from build123d import *

# Parameters (mm, degrees)
SKETCH1_W                       = 82.55
SKETCH1_H                       = 57.15
BOSS_EXTRUDE1_DEPTH             = 8.636
FILLET2_R                       = 7.62
FILLET3_R                       = 3.81
SKETCH2_W                       = 63.5
SKETCH2_H                       = 40.64
CUT_EXTRUDE1_DEPTH              = 5.461
SKETCH7_W                       = 68.58
SKETCH7_H                       = 45.72
BOSS_EXTRUDE3_DEPTH             = 5.08
SKETCH8_W                       = 63.5
SKETCH8_H                       = 40.64
CUT_EXTRUDE3_DEPTH              = 5.08
SKETCH5_R                       = 1.016
BOSS_EXTRUDE4_DEPTH             = 12.7
SKETCH4_R                       = 2.25
SKETCH4_W                       = 12.6
SKETCH4_H                       = 5
SKETCH4_W_2                     = 6.604
SKETCH4_H_2                     = 6.604
CUT_EXTRUDE2_DEPTH              = 7.366
FILLET7_R                       = 1.016
FILLET8_R                       = 2.54
SKETCH9_W                       = 12.753817634
SKETCH9_H                       = 4.826
BOSS_EXTRUDE5_DEPTH             = 5.08
FILLET10_R                      = 7.62
FILLET11_R                      = 1.27
FILLET12_R                      = 1.016
F_4_40_TAPPED_HOLE2_D           = 2.2606
F_4_40_TAPPED_HOLE2_DEPTH       = 7.62
F_4_40_TAPPED_HOLE2_CSINK_D     = 4.1148
F_4_40_TAPPED_HOLE2_CSINK_ANGLE = 100
F_4_40_TAPPED_HOLE2_TIP         = 0.679152758


with BuildPart() as part:
    # Sketch1 → Boss-Extrude1 (new body)
    with BuildSketch(Plane(origin=(0, 0, 0), x_dir=(1, 0, 0), z_dir=(0, 1, 0))):
        with Locations((41.275, 28.575)):
            Rectangle(SKETCH1_W, SKETCH1_H)
    extrude(amount=BOSS_EXTRUDE1_DEPTH)

    # Fillet2
    fillet2_edges = [part.edges().sort_by_distance(p)[0] for p in [
        (0, 4.318, -57.15),
        (82.55, 4.318, -57.15),
        (82.55, 4.318, 0),
        (0, 4.318, 0),
    ]]
    fillet(fillet2_edges, radius=FILLET2_R)

    # Fillet3
    fillet3_edges = [part.edges().sort_by_distance(p)[0] for p in [
        (41.275, 0, -57.15),
        (0, 0, -28.575),
        (82.55, 0, -28.575),
        (41.275, 0, 0),
        (2.231846327, 0, -54.918153673),
        (2.231846327, 0, -2.231846327),
        (80.318153673, 0, -2.231846327),
        (80.318153673, 0, -54.918153673),
    ]]
    fillet(fillet3_edges, radius=FILLET3_R)

    # Sketch2 → Cut-Extrude1 (cut)
    with BuildSketch(Plane(origin=(0, 8.636, 0), x_dir=(1, 0, 0), z_dir=(0, 1, 0))):
        with Locations((41.275, 28.575)):
            Rectangle(SKETCH2_W, SKETCH2_H)
    extrude(amount=-CUT_EXTRUDE1_DEPTH, mode=Mode.SUBTRACT)

    # Sketch7 → Boss-Extrude3 (add)
    with BuildSketch(Plane(origin=(0, 8.636, 0), x_dir=(1, 0, 0), z_dir=(0, 1, 0))):
        with Locations((41.275, 28.575)):
            Rectangle(SKETCH7_W, SKETCH7_H)
    extrude(amount=BOSS_EXTRUDE3_DEPTH)

    # Sketch8 → Cut-Extrude3 (cut)
    with BuildSketch(Plane(origin=(0, 13.716, 0), x_dir=(1, 0, 0), z_dir=(0, 1, 0))):
        with Locations((41.275, 28.575)):
            Rectangle(SKETCH8_W, SKETCH8_H)
    extrude(amount=-CUT_EXTRUDE3_DEPTH, mode=Mode.SUBTRACT)

    # Sketch5 → Boss-Extrude4 (add)
    with BuildSketch(Plane(origin=(0, 3.175, 0), x_dir=(1, 0, 0), z_dir=(0, 1, 0))):
        with Locations(Location((17.665, 42.392, 0), (0, 0, 90))):
            Circle(SKETCH5_R)
        with Locations(Location((17.665, 14.732, 0), (0, 0, 90))):
            Circle(SKETCH5_R)
        with Locations(Location((67.945, 42.259, 0), (0, 0, 90))):
            Circle(SKETCH5_R)
        with Locations(Location((67.945, 14.859, 0), (0, 0, 90))):
            Circle(SKETCH5_R)
    extrude(amount=BOSS_EXTRUDE4_DEPTH)

    # Sketch4 → Cut-Extrude2 (cut)
    with BuildSketch(Plane(origin=(0, 3.175, 0), x_dir=(1, 0, 0), z_dir=(0, 1, 0))):
        with Locations(Location((45.641, 18.034, 0), (0, 0, 270))):
            Circle(SKETCH4_R)
        with Locations((60.171, 18.059)):
            Rectangle(SKETCH4_W, SKETCH4_H)
        with Locations((32.983, 18.034)):
            Rectangle(SKETCH4_W_2, SKETCH4_H_2)
    extrude(amount=-CUT_EXTRUDE2_DEPTH, mode=Mode.SUBTRACT)

    # Fillet7
    fillet7_edges = [part.edges().sort_by_distance(p)[0] for p in [
        (17.665, 15.875, -41.376),
        (17.665, 15.875, -13.716),
        (67.945, 15.875, -41.243),
    ]]
    fillet(fillet7_edges, radius=FILLET7_R)

    # Fillet8
    fillet8_edges = [part.edges().sort_by_distance(p)[0] for p in [
        (75.565, 11.176, -51.435),
        (6.985, 11.176, -51.435),
        (6.985, 11.176, -5.715),
        (75.565, 11.176, -5.715),
    ]]
    fillet(fillet8_edges, radius=FILLET8_R)

    # Sketch9 → Boss-Extrude5 (add)
    with BuildSketch(Plane.XY):
        with Locations((41.275, 6.223)):
            Rectangle(SKETCH9_W, SKETCH9_H)
    extrude(amount=BOSS_EXTRUDE5_DEPTH)

    # Fillet10
    # the kernel refuses this fillet: 7.62 mm, written as the material it takes off along each edge
    with BuildSketch(Plane(origin=(47.651908817, -14.150512242, 5.08), x_dir=(0, 0, -1), z_dir=(0, 1, 0)), Plane(origin=(34.898091183, 26.596512242, 5.08), x_dir=(0, 0, -1), z_dir=(0, -1, 0))) as fillet10_piece_1:
        with BuildLine():
            CenterArc((7.62, 7.184204897), FILLET10_R, 180, 70.528779366)
            Line((0, 7.184204897), (-0.1524, 7.184204897))
            Line((-0.1524, 7.184204897), (-0.1524, 0))
            Line((-0.1524, 0), (0, -0.1524))
            ThreePointArc((0, -0.1524), (2.54, -0.1524), (5.0292, -0.143684098))
            Line((5.0292, -0.143684098), (5.08, 0))
        make_face()
    extrude(amount=40.747024484, mode=Mode.SUBTRACT)

    # Fillet11
    fillet11_edges = [part.edges().sort_by_distance(p)[0] for p in [
        (41.275, 13.716, -51.435),
        (75.565, 13.716, -28.575),
        (6.985, 13.716, -28.575),
        (41.275, 13.716, -5.715),
        (7.728948776, 13.716, -50.691051224),
        (7.728948776, 13.716, -6.458948776),
        (74.821051224, 13.716, -6.458948776),
        (74.821051224, 13.716, -50.691051224),
    ]]
    fillet(fillet11_edges, radius=FILLET11_R)

    # Fillet12
    fillet12_edges = [part.edges().sort_by_distance(p)[0] for p in [
        (67.945, 15.875, -13.843),
    ]]
    fillet(fillet12_edges, radius=FILLET12_R)

    # #4-40 Tapped Hole2
    with Locations(Plane(origin=(0, 3.81, 0), x_dir=(-1, 0, 0), z_dir=(0, -1, 0))):
        with Locations((-41.275, -2.518557543)):
            CounterSinkHole(F_4_40_TAPPED_HOLE2_D / 2, F_4_40_TAPPED_HOLE2_CSINK_D / 2, depth=F_4_40_TAPPED_HOLE2_DEPTH, counter_sink_angle=F_4_40_TAPPED_HOLE2_CSINK_ANGLE)
            with Locations((0, 0, -(F_4_40_TAPPED_HOLE2_DEPTH + F_4_40_TAPPED_HOLE2_TIP / 2))):  # 118° drill point
                Cone(0, F_4_40_TAPPED_HOLE2_D / 2, F_4_40_TAPPED_HOLE2_TIP, mode=Mode.SUBTRACT)


solid = part.part
The listing builds one solid part. Answer for the finished solid, in the listing's coordinates (mm). A direction names the side the tool comes from. Give positions to 0.01 mm unless a question says otherwise; leave off trailing zeros. Write each loop counter-clockwise with the first axis right and the second up, starting at its lowest first coordinate (ties: lowest second). Pieces come first, ordered by that corner, then holes.
1) A tool of negligible diameter and unlimited length cuts with its end or side. For faces 4 (the face through (33, 2, -21.336)), 5 (the face through (41, 11, -5.715)), 6 (the face through (7.71, 10.57, -6.48)), 7 (the face through (74.8, 10.57, -6.44)), 8 (the face through (67.64, 8.94, -15.83)), from which of +Z, -Z, +X, -X, +Y, -Y can it reach the whole face along a straight path? Write none if from no direction.
2) For a pull along X with two mould halves and no side action, classify faces 1 (the face through (73.025, 9, -28)), 2 (the face through (0, 6, -28)), 3 (the face through (74.8, 10.57, -50.71)) as pulls with the +X half, pulls with the -X half, needs draft (parallel to the pull), parting line crosses it, or undercut.
3) Section A-A (x = 12.5) is taken. Write down the section's boundary in (y, z) (3 decimals).
4) Find the intervals of material crossed by L1, parallel to X at y = 6.75, z = -39 (3 decimals); L2, parallel to X at y = 11, z = -18 (3 decimals); L3, parallel to Z at x = 26.5, y = 12 (3 decimals), in increasing order.
5) Section C-C (z = -9.5) is taken. Write down the section's boundary in (x, y) (3 decimals), and give its area (3 significant figures).
6) Given P1, Ø1, axis at x = 33, y = 2, coming from the +Z side; P2, Ø5, axis at y = 14, z = -49.5, coming from the -X side (3 decimals); P3, Ø2.5, axis at x = 39, z = 2, coming from the -Y side; P4, Ø1.4, axis at x = 41.28, z = 2.52, coming from the -Y side, each flat-ended and moving along its own axis, determine where each tip first touches the part or whether it passes through.
7) Section B-B (y = 7.25) is taken. Write down the section's boundary in (x, z) (3 decimals), and give its area (3 significant figures).
Response:
1. face 4: +Y, -Y
1. face 5: +Z, +X, -X, +Y
1. face 6: +Z, -X, +Y
1. face 7: +Z, +X, +Y
1. face 8: +Y
2. face 1: undercut
2. face 2: pulls with the -X half
2. face 3: pulls with the +X half
3. outline: (0, -53.34) arc R3.81 ccw to (3.81, -57.15) - (8.636, -57.15) - (8.636, -51.435) - (12.446, -51.435) arc R1.27 ccw to (13.716, -50.165) - (13.716, -48.895) - (3.175, -48.895) - (3.175, -8.255) - (13.716, -8.255) - (13.716, -6.985) arc R1.27 ccw to (12.446, -5.715) - (8.636, -5.715) - (8.636, 0) - (3.81, 0) arc R3.81 ccw to (0, -3.81) - close
4. L1: x = 0 to 9.525, 73.025 to 82.55
4. L2: x = 6.985 to 9.525, 73.025 to 75.565
4. L3: z = -51.435 to -48.895, -8.255 to -5.715
5. outline: (0, 3.81) arc R3.81 ccw to (3.81, 0) - (78.74, 0) arc R3.81 ccw to (82.55, 3.81) - (82.55, 8.636) - (75.565, 8.636) - (75.565, 12.446) arc R1.27 ccw to (74.295, 13.716) - (73.025, 13.716) - (73.025, 3.175) - (9.525, 3.175) - (9.525, 13.716) - (8.255, 13.716) arc R1.27 ccw to (6.985, 12.446) - (6.985, 8.636) - (0, 8.636) - close
5. area: 385 mm2
6. P1: stops at z = -0.23
6. P2: stops at x = 6.985
6. P3: stops at y = 3.81
6. P4: passes through
7. outline: (0, -49.53) arc R7.62 ccw to (7.62, -57.15) - (74.93, -57.15) arc R7.62 ccw to (82.55, -49.53) - (82.55, -7.62) arc R7.62 ccw to (74.93, 0) - (47.652, 0) arc R7.62 ccw to (41.275, 5.037) arc R7.62 ccw to (34.898, 0) - (7.62, 0) arc R7.62 ccw to (0, -7.62) - close; circle Ø2.032 at (17.665, -42.392); circle Ø2.032 at (17.665, -14.732); circle Ø2.032 at (67.945, -42.259); circle Ø2.032 at (67.945, -14.859); hole (9.525, -48.895) - (73.025, -48.895) - (73.025, -8.255) - (9.525, -8.255) - close; hole circle Ø2.261 at (41.275, 2.519)
7. area: 2,140 mm2
